Check sheet for the modelled part. Datum: model origin and axes. Units: mm. Give positions to 0.01 mm unless a question says otherwise; leave off trailing zeros. Loops run counter-clockwise (first coordinate to the right, second up) from the corner with the lowest first, then second, coordinate; pieces in that order, holes last. Notation, with made-up numbers: M -36,41 L -18,41 A25 cw -18,75 Z; hole C 74.25,15 d4. An arc over 180 degrees is marked long. Put each result on its own line as item: value. Start each with the question number.
```python
from build123d import *

# Parameters (mm, degrees)
F2_R        = 1.25
F3_DEPTH    = 20.848816548
F4_T2_ANGLE = 269.9999999999
F4_T4_ANGLE = 90.0000002223


# Not quite as in the source:
# - a fillet or chamfer that OpenCascade refuses, or shapes differently, is made with other operations: its cross-section is extruded or revolved along the edge and cut away or added


with BuildPart() as f1:
    # F0 (on Front) → F1 (revolve)
    with BuildSketch(Plane.XZ):
        with BuildLine():
            ThreePointArc((20.847816448, 19.2961636657), (20.2143632876, 20.8119613812), (18.6907213238, 21.4263072013))
            ThreePointArc((18.6907213238, 21.4263072013), (16.8507396209, 20.3225249849), (16.9045229372, 18.1775365926))
            ThreePointArc((16.9045229372, 18.1775365926), (19.2988876007, 17.2467192141), (20.847816448, 19.2961636657))
        make_face()
        with BuildLine():
            Line((-1.75, 5.5), (0, 5.5))
            Line((0, 5.5), (0, 0))
            Line((0, 0), (0.6667277431, 0))
            ThreePointArc((0.6667277431, 0), (5.3173187467, 12.1869687509), (16.9045229372, 18.1775365926))
            ThreePointArc((16.9045229372, 18.1775365926), (16.8507396209, 20.3225249849), (18.6907213238, 21.4263072013))
            ThreePointArc((18.6907213238, 21.4263072013), (5.7901979365, 16.9030256739), (-1.75, 5.5))
        make_face()
    revolve(axis=Axis((0.3358235447, 0, 0), (1, 0, 0)))

    # F2 (on face) → F3 (cut, through all)
    with BuildSketch(Plane(origin=(0, 0, 0), x_dir=(0, -1, 0), z_dir=(-1, 0, 0))):
        Circle(F2_R)
    extrude(amount=-F3_DEPTH, mode=Mode.SUBTRACT)

    # F4: chamfer of 0.5 on 2 edges, made by hand

    # F4_s1 → F4_t2 (revolve, cut)
    with BuildSketch(Plane.XZ):
        with BuildLine():
            Line((0.7639536686, 1.7481015134), (0.2013545471, 1.2365450652))
            Line((0.2013545471, 1.2365450652), (0.2013545471, 1.2265450652))
            ThreePointArc((0.2013545471, 1.2265450652), (0.4554194631, 1.24), (0.7094843791, 1.24))
            Line((0.7094843791, 1.24), (0.7194610064, 1.2493166933))
            ThreePointArc((0.7194610064, 1.2493166933), (0.7382742313, 1.4989228259), (0.7739086095, 1.7471532769))
            Line((0.7739086095, 1.7471532769), (0.7639536686, 1.7481015134))
        make_face()
    revolve(axis=Axis((0.7094843791, 0, 0), (-1, 0, 0)), revolution_arc=F4_T2_ANGLE, mode=Mode.SUBTRACT)

    # F4_s3 → F4_t4 (revolve, cut)
    with BuildSketch(Plane.XY.offset(2.5e-09)):
        with BuildLine():
            Line((0.7639536686, -1.7481015124), (0.2013545471, -1.2365450642))
            Line((0.2013545471, -1.2365450642), (0.2013545471, -1.2265450642))
            ThreePointArc((0.2013545471, -1.2265450642), (0.4554194631, -1.239999999), (0.7094843791, -1.24))
            Line((0.7094843791, -1.24), (0.7194610064, -1.2493166933))
            ThreePointArc((0.7194610064, -1.2493166933), (0.7382742313, -1.4989228254), (0.7739086095, -1.7471532759))
            Line((0.7739086095, -1.7471532759), (0.7639536686, -1.7481015124))
        make_face()
    revolve(axis=Axis((0.7094843791, -2.4e-09, 2.5e-09), (-1, 0, 0)), revolution_arc=F4_T4_ANGLE, mode=Mode.SUBTRACT)


solid = f1.part
```
Q1. Depth check by flat-ended pin: P1, Ø5, axis at y = -2.5, z = -8.5, coming from the -X side; P2, Ø3, axis at y = 0, z = 0, coming from the +X side; P3, Ø4, axis at y = -1, z = -0.5, coming from the +X side. Enter the tip coordinate at first touch or a pass-through.
Q2. Thickness scan on line 1 along Z through (x, y) = (6.75, -6); line 2 along Z through (x, y) = (0.2, 0); line 3 along Y through (x, z) = (0.25, 0). Record the ranges inside material, lowest first. Write a range as [from, to].
Q3. Section check A-A, the plane x = 1.5. Record the cut outline in (y, z).
Found:
1. P1: stops at x = -1.5
1. P2: stops at x = 0.49
1. P3: stops at x = 0.93
2. line 1: z = [-16.56, -12.23], [12.23, 16.56]
2. line 2: z = [-10.35, -1.25], [1.25, 10.35]
2. line 3: y = [-10.44, -1.28], [1.28, 10.44]
3. outline: C 0,0 d24.84; hole C 0,0 d10.92
